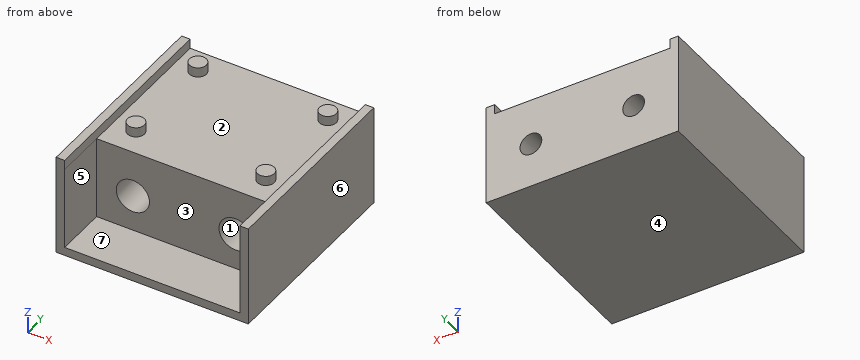
```python
from build123d import *

# Parameters (mm, degrees)
SKETCH_W        = 31.8
SKETCH_H        = 33.4
PAD_DEPTH       = 15.1
SKETCH001_R     = 1.4
SKETCH001_W     = 1.4
SKETCH001_H     = 33.4
PAD001_DEPTH    = 1.6
SKETCH002_W     = 29
SKETCH002_H     = 13.7
POCKET_DEPTH    = 8.5
SKETCH011_R     = 2.75
POCKET006_DEPTH = 8
SKETCH012_R     = 1.8
POCKET007_DEPTH = 20


with BuildPart() as part:
    # Sketch (on Face1449 of Binder) → Pad (new body)
    with BuildSketch(Plane(origin=(0, 0, 0), x_dir=(1, 0, 0), z_dir=(0, 0, -1))):
        with Locations((13.749781, -17.25)):
            Rectangle(SKETCH_W, SKETCH_H)
    extrude(amount=PAD_DEPTH)

    # Sketch001 (on Face5 of Pad) → Pad001 (join)
    with BuildSketch(Plane.XY):
        with Locations((3, 30)):
            Circle(SKETCH001_R)
        with Locations((24.5, 30)):
            Circle(SKETCH001_R)
        with Locations((3, 13.5)):
            Circle(SKETCH001_R)
        with Locations((24.5, 13.5)):
            Circle(SKETCH001_R)
        with Locations((-1.450219, 17.25)):
            Rectangle(SKETCH001_W, SKETCH001_H)
        with Locations((28.949781, 17.25)):
            Rectangle(SKETCH001_W, SKETCH001_H)
    extrude(amount=PAD001_DEPTH)

    # Sketch002 (on Face16 of Pad001) → Pocket (cut)
    with BuildSketch(Plane.XZ.offset(-0.55)):
        with Locations((13.74978, -6.85)):
            Rectangle(SKETCH002_W, SKETCH002_H)
    extrude(amount=-POCKET_DEPTH, mode=Mode.SUBTRACT)

    # Sketch011 (on Face10 of Pocket) → Pocket006 (cut)
    with BuildSketch(Plane.XZ.offset(-9.05)):
        with Locations((5.24978, -7.7)):
            Circle(SKETCH011_R)
        with Locations((22.24978, -7.7)):
            Circle(SKETCH011_R)
    extrude(amount=-POCKET006_DEPTH, mode=Mode.SUBTRACT)

    # Sketch012 (on Face19 of Pocket006) → Pocket007 (cut)
    with BuildSketch(Plane.XZ.offset(-17.05)):
        with Locations((5.24978, -7.7)):
            Circle(SKETCH012_R)
        with Locations((22.24978, -7.7)):
            Circle(SKETCH012_R)
    extrude(amount=-POCKET007_DEPTH, mode=Mode.SUBTRACT)


solid = part.part
```
Check sheet for the modelled part. Datum: model origin and axes. Units: mm. Face numbers are marked on the shaded views. A direction names the side the tool comes from. Give positions to 0.01 mm unless a question says otherwise; leave off trailing zeros. Order: outer loops, then holes, each group sorted by start corner. A loop starts at its lowest first (then second) coordinate and runs counter-clockwise, first axis right, second up. Notation, with made-up numbers: M 63.5,-32.5 L 117.5,-32.5 A34 cw 117.5,6.5 Z; hole C 13.5,68 d4. An arc over 180 degrees is marked long. Answer in a Markdown table with one row per item.
1) Release check for a two-part mould opening along X. For the marked faces 4, 5, 6 and 7 record: +X half, -X half, draft (parallel to the pull), parting line (faces both ways), or undercut.
Filled sheet:
| item | result |
|---|---|
| face 4 | draft |
| face 5 | undercut |
| face 6 | +X half |
| face 7 | undercut |
2) Cross-section at A-A, the plane y = 19. Enter the section's corners in (x, z), plus the area to 3 significant figures.
Filled sheet:
| item | result |
|---|---|
| outline | M -2.15,-15.1 L 29.65,-15.1 L 29.65,1.6 L 28.25,1.6 L 28.25,0 L -0.75,0 L -0.75,1.6 L -2.15,1.6 Z; hole C 5.25,-7.7 d3.6; hole C 22.25,-7.7 d3.6 |
| area | 464 mm2 |
3) Thickness scan on L1, parallel to X at y = 4.5, z = -12.75; L2, parallel to X at y = 16.5, z = -8; L3, parallel to X at y = 19.5, z = -6.5. Record the ranges inside material, lowest first. Write a range as [from, to].
Filled sheet:
| item | result |
|---|---|
| L1 | x = [-2.15, -0.75], [28.25, 29.65] |
| L2 | x = [-2.15, 2.52], [7.98, 19.52], [24.98, 29.65] |
| L3 | x = [-2.15, 3.91], [6.59, 20.91], [23.59, 29.65] |
4) Gauge pin test, flat ends, axial feed: P1, Ø3, axis at x = 17.5, z = -0.5, coming from the -Y side; P2, Ø2, axis at x = 7, y = 18.5, coming from the +Z side; P3, Ø2.5, axis at x = 18.5, y = 5.5, coming from the +Z side. Record the tip position at first contact, or that the pin passes through.
Filled sheet:
| item | result |
|---|---|
| P1 | stops at y = 9.05 |
| P2 | stops at z = 0 |
| P3 | stops at z = -13.7 |
5) Access from +Z, -Z, +X, -X, +Y, -Y to the whole of each face (thin tool, end or side, straight path). Record for the marked faces 1, 2 and 3.
Filled sheet:
| item | result |
|---|---|
| face 1 | -Y |
| face 2 | +Z |
| face 3 | +Z, -Y |
6) Cross-section at D-D, the plane z = -1.75. Enter the section's corners in (x, y), plus the area to 3 significant figures.
Filled sheet:
| item | result |
|---|---|
| outline | M -2.15,0.55 L -0.75,0.55 L -0.75,9.05 L 28.25,9.05 L 28.25,0.55 L 29.65,0.55 L 29.65,33.95 L -2.15,33.95 Z |
| area | 816 mm2 |
7) Cross-section at B-B, the plane z = -7.7. Enter the section's corners in (x, y).
Filled sheet:
| item | result |
|---|---|
| outline | M -2.15,0.55 L -0.75,0.55 L -0.75,9.05 L 2.5,9.05 L 2.5,17.05 L 3.45,17.05 L 3.45,33.95 L -2.15,33.95 Z; M 7.05,17.05 L 8,17.05 L 8,9.05 L 19.5,9.05 L 19.5,17.05 L 20.45,17.05 L 20.45,33.95 L 7.05,33.95 Z; M 24.05,17.05 L 25,17.05 L 25,9.05 L 28.25,9.05 L 28.25,0.55 L 29.65,0.55 L 29.65,33.95 L 24.05,33.95 Z |
